Autodesk Inventor part; units mm, degrees
ref_plane "YZ Plane" through (0, 0, 0) normal (1, 0, 0) x (0, 1, 0)
ref_plane "XZ Plane" through (0, 0, 0) normal (0, 1, 0) x (-1, 0, 0)
ref_plane "XY Plane" through (0, 0, 0) normal (0, 0, 1) x (1, 0, 0)
sketch "Sketch1" plane through (0, 0, 0) normal (0, 0, 1) x (1, 0, 0)
  line L0 (0, 75) -> (33, 75)
  line L1 (33, 75) -> (33, 67)
  line L2 (33, 67) -> (0, 67)
  line L3 (0, 67) -> (0, 75)
  line L4 (14.75, 67) -> (15.75, 68)
  line L5 (15.75, 68) -> (17.25, 68)
  line L6 (17.25, 68) -> (18.25, 67)
  line L7 (15.25, 67.5) -> (17.75, 67.5)
  line L8 (17.75, 67.5) -> (17.75, 67)
  line L9 (17.75, 67) -> (15.25, 67)
  line L10 (15.25, 67) -> (15.25, 67.5)
  circle A0 centre (22, 65.5) radius 2
  line L11 (0, -15) -> (0, 90)
  line L12 (-6.6, 0) -> (39.6, 0)
  point P0 (0, 0)
  point P1 (20, 65.5)
  point P2 (16.5, 68)
  point P3 (16.5, 67)
  point P4 (20.6771, 67)
  point P5 (23.3229, 67)
  dimension "d7" = 4
  dimension "d0" = 2.5
  dimension "d1" = 67.5
  dimension "d2" = 0.5
  dimension "d3" = 75
  dimension "d4" = 1
  dimension "d5" = 33
  dimension "d8" = 1.75
  dimension "d10" = 67
revolve "Revolution1" add sketch "Sketch1" angle 360 about axis through (-10, 0, 0) along (1, 0, 0) contours L0 L1 L2 A0 L6 L5 L4 L3
properties part number "One Piece Ring" material "UHMW, Black"
Geometry check sheet. Reference: the model listing, model coordinates, mm. Give positions to 0.01 mm unless a question says otherwise; leave off trailing zeros. Write each loop counter-clockwise with the first axis right and the second up, starting at its lowest first coordinate (ties: lowest second). Pieces come first, ordered by that corner, then holes. Notation, with made-up numbers: M -6.5,-22.5 L 3.5,-22.5 A11 ccw 3.5,-7.5 Z; hole C -22,24 d9. An arc over 180 degrees is marked long. One line per question, with ' | ' between items.
1. Mould release check, pull along X, two halves, no side actions. Record for faces 1 (the face through (33, -28.1, 61.5)), 2 (the face through (28.094, -14.524, 65.407)), 3 (the face through (16.51, 36.556, 57.338)), 4 (the face through (0, -28.1, 61.5)): released by +X, released by -X, zero draft, split by the parting line, or undercut.
Ans:
face 1: released by +X | face 2: zero draft | face 3: undercut | face 4: released by -X
2. Scan lines: line 1 along Z through (x, y) = (16.1, 0); line 2 along Z through (x, y) = (11.75, 0); line 3 along Y through (x, z) = (23, -39). Record each from-to range of solid material in increasing order. Write a range as from..to.
Ans:
line 1: -75..-68, 68..75 | line 2: -75..-67, 67..75 | line 3: -64.06..-54.76, 54.76..64.06
3. Cross-section at C-C (x = 13). Enter the section's corners in (y, z).
Ans:
outline: C 0,0 d150; hole C 0,0 d134
4. Gauge pin test, flat ends, axial feed: pin 1 (5 mm diameter, centred on x = 16.5, z = 16.5, fed in from -Y); pin 2 (1.5 mm diameter, centred on x = 8, y = -16.5, fed in from -Z); pin 3 (12 mm diameter, centred on x = 25.5, y = 16, fed in from -Z). Record the tip position at first contact, or that the pin passes through.
Ans:
pin 1: y = -73.68 | pin 2: z = -73.33 | pin 3: z = -74.33
5. Cross-section at A-A (y = 0). Enter the section's corners in (x, z), plus the area to 3 significant figures.
Ans:
outline: M 0,-75 L 33,-75 L 33,-67 L 23.32,-67 A2 cw 20.68,-67 L 18.25,-67 L 17.25,-68 L 15.75,-68 L 14.75,-67 L 0,-67 Z; M 0,67 L 14.75,67 L 15.75,68 L 17.25,68 L 18.25,67 L 20.68,67 A2 cw 23.32,67 L 33,67 L 33,75 L 0,75 Z | area: 521 mm2
